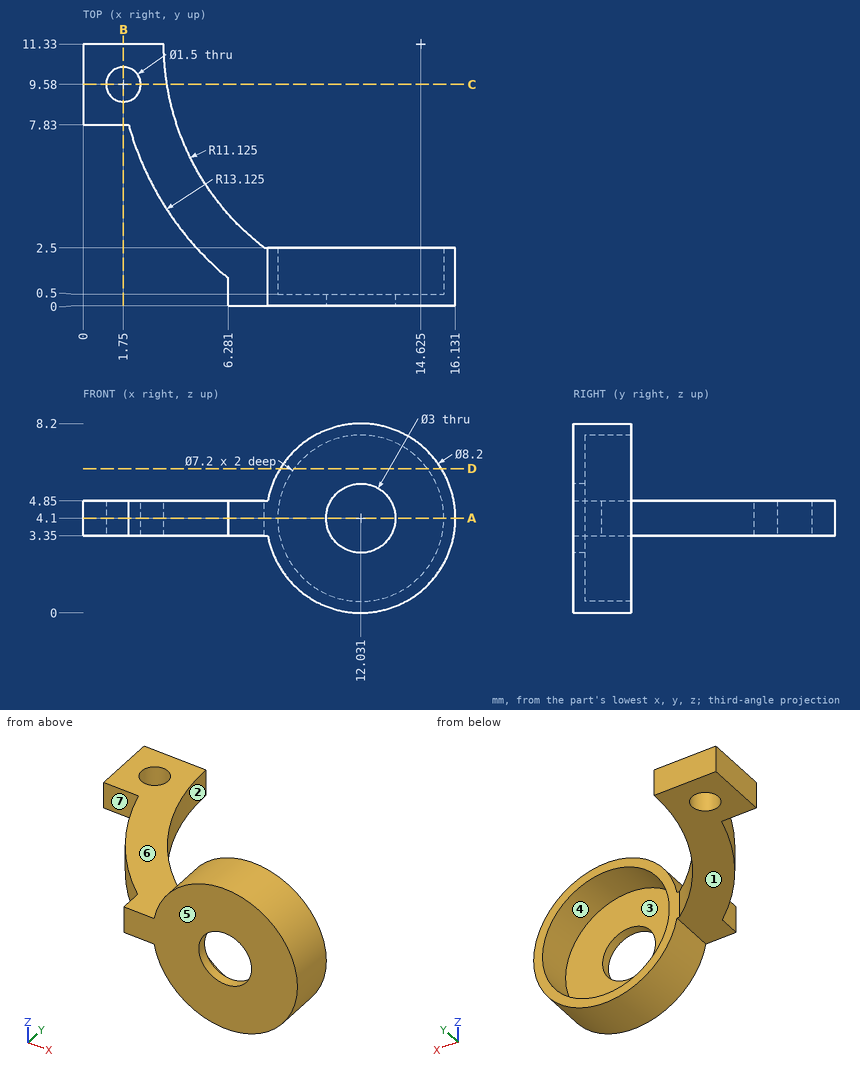
For this review, use the dimensioned drawing (mm, ordinates from the lowest corner) and the shaded views. A direction names the side the tool comes from. Coordinates: 2 decimals unless noted, no trailing zeros. Order: outer loops, then holes, each group sorted by start corner. A loop starts at its lowest first (then second) coordinate and runs counter-clockwise, first axis right, second up. Notation, with made-up numbers: (-23, 69) - (-14, 69) arc R21 ccw to (-14, 85) - close; hole circle Ø4 at (49.5, -37). An arc over 180 degrees is marked (long way). Answer as a JSON object with one key per item and string values. Group by question number.
1. We need section C-C on y = 9.58. State the section outline as (x, z) points.
2. For the marked faces 5, 6 and 7, list the 3-axis set-ups (+Z, -Z, +X, -X, +Y, -Y) from which the entire face can be reached by the end or side of a thin tool; tool diameter is ignored.
3. The part is to be moulded in two halves that separate along Z. For the marked faces 1, 2, 3 and 4, say which applies: pulls with the +Z half, pulls with the -Z half, needs draft (parallel to the pull), parting line crosses it, or undercut.
4. We need section A-A on z = 4.1. Give the number of separate pieces and of enclosed holes in the cut face.
5. We need section D-D on z = 6.25. State the section outline as (x, y) points.
6. For probe 1 along Y at (x, z) = (1.75, 3.75); probe 2 along Y at (x, z) = (10, 3.75); probe 3 along X at (y, z) = (2.25, 7) (1 decimal), list the stretches that pass through material, from the lowest coordinate up.
7. We need section B-B on x = 1.75. State the section outline as (y, z) points.
8. Clearance check with flat-ended pins moving along their axes: P1, Ø1.5, axis at x = 3.5, y = 8, coming from the -Z side; P2, Ø2, axis at x = 4, z = 5, coming from the -Y side; P3, Ø0.6, axis at y = 1, z = 4, coming from the -X side. State where each tip first meets the part, or that it passes through.
Final values:
{
 "1": {"outline": "(0, 3.35) - (1, 3.35) - (1, 4.85) - (0, 4.85) - close; (2.5, 3.35) - (3.64, 3.35) - (3.64, 4.85) - (2.5, 4.85) - close"},
 "2": {"face 5": "+Z, -Z, +X, -X, -Y", "face 6": "+Z, -X, +Y, -Y", "face 7": "+Z, -Z, -X, -Y"},
 "3": {"face 1": "pulls with the -Z half", "face 2": "needs draft", "face 3": "undercut", "face 4": "undercut"},
 "4": {"separate pieces": "2", "enclosed holes": "1"},
 "5": {"outline": "(8.54, 0) - (15.52, 0) - (15.52, 2.5) - (14.92, 2.5) - (14.92, 0.5) - (9.14, 0.5) - (9.14, 2.5) - (8.54, 2.5) - close"},
 "6": {"probe 1": "7.83 to 8.83, 10.33 to 11.33", "probe 2": "0 to 0.5", "probe 3": "9.1 to 9.9, 14.2 to 14.9"},
 "7": {"outline": "(7.83, 3.35) - (8.83, 3.35) - (8.83, 4.85) - (7.83, 4.85) - close; (10.33, 3.35) - (11.33, 3.35) - (11.33, 4.85) - (10.33, 4.85) - close"},
 "8": {"P1": "z = 3.35", "P2": "y = 2.42", "P3": "x = 6.16"}
}
